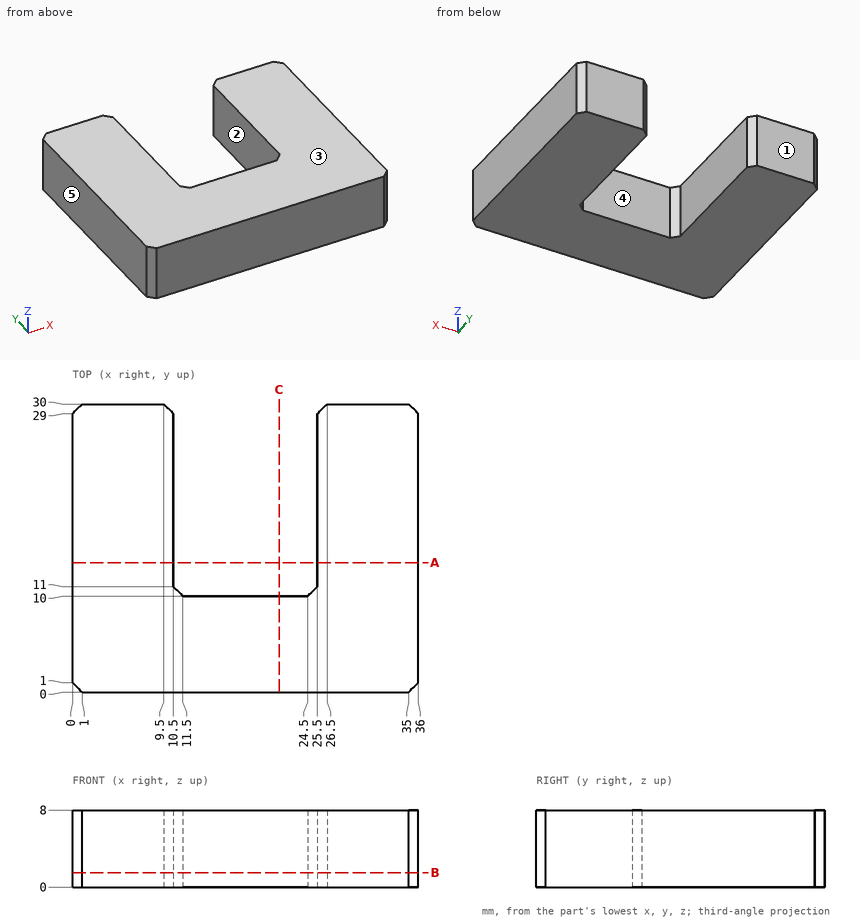
Verification items for this drawing (mm, ordinates from the low corner). A direction names the side the tool comes from. Give positions to 0.01 mm unless a question says otherwise; leave off trailing zeros. Loops run counter-clockwise (first coordinate to the right, second up) from the corner with the lowest first, then second, coordinate; pieces in that order, holes last. Notation, with made-up numbers: M -32,-21 L -22,-21 A34 cw -22,18 Z; hole C 64.5,41 d3. An arc over 180 degrees is marked long. Answer as a JSON object with one key per item and string values. Group by question number.
Q1. Release check for a two-part mould opening along X. For the marked faces 3, 4 and 5 record: released by +X, released by -X, zero draft, split by the parting line, or undercut.
Q2. Cross-section at C-C on x = 21.5. Record the cut outline in (y, z), then the cut area to 3 significant figures.
Q3. Cross-section at B-B on z = 1.5. Record the cut outline in (x, y).
Q4. Access from +Z, -Z, +X, -X, +Y, -Y to the whole of each face (thin tool, end or side, straight path). Record for the marked faces 1 and 2.
Q5. Go/stop test with a flat-tipped pin: P1, Ø4, axis at x = 17.5, z = 3, coming from the +Y side. Record where the tip stops, or that it passes through.
Q6. Material ranges on line 1 along X through (y, z) = (27.25, 1.75); line 2 along Y through (x, z) = (21, 2.75); line 3 along X through (y, z) = (10.5, 7), recorded low to high. Write a range as [from, to].
Q7. Cross-section at A-A on y = 13.5. Record the cut outline in (x, z).
Evaluation:
{
 "1": {"face 3": "zero draft", "face 4": "undercut", "face 5": "released by -X"},
 "2": {"outline": "M 0,0 L 10,0 L 10,8 L 0,8 Z", "area": "80.0 mm2"},
 "3": {"outline": "M 0,1 L 1,0 L 35,0 L 36,1 L 36,29 L 35,30 L 26.5,30 L 25.5,29 L 25.5,11 L 24.5,10 L 11.5,10 L 10.5,11 L 10.5,29 L 9.5,30 L 1,30 L 0,29 Z"},
 "4": {"face 1": "+Z, -Z, +X, -X, +Y", "face 2": "+Z, -Z, +Y"},
 "5": {"P1": "stops at y = 10"},
 "6": {"line 1": "x = [0, 10.5], [25.5, 36]", "line 2": "y = [0, 10]", "line 3": "x = [0, 11], [25, 36]"},
 "7": {"outline": "M 0,0 L 10.5,0 L 10.5,8 L 0,8 Z; M 25.5,0 L 36,0 L 36,8 L 25.5,8 Z"}
}
